For this review, take the finished solid that the model builds, in its own axes (mm). Face numbers are marked on the shaded views. A direction names the side the tool comes from. Round coordinates to 2 decimals unless told otherwise and drop trailing zeros. Write each loop counter-clockwise with the first axis right and the second up, starting at its lowest first coordinate (ties: lowest second). Pieces come first, ordered by that corner, then holes. Notation, with made-up numbers: M 28.5,49.5 L 78.5,49.5 A20 cw 78.5,88.5 Z; hole C 0,-24.75 d9. An arc over 180 degrees is marked long. Answer in a Markdown table with one row per item.
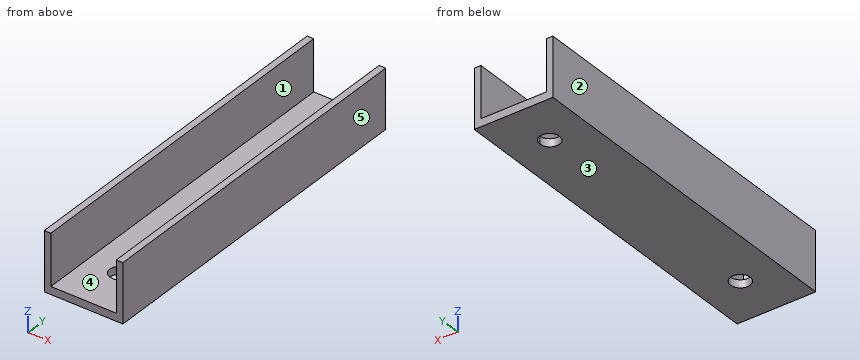
```python
from build123d import *

# Parameters (mm, degrees)
F0_R     = 3.175
F1_DEPTH = 19.05
F2_W     = 21.134718
F2_H     = 23.147546
F3_DEPTH = 140.54349


with BuildPart() as f1:
    # F0 (on Top) → F1 (new body)
    with BuildSketch(Plane.XY):
        with BuildLine():
            ThreePointArc((3.175, 41.452094), (2.245064, 43.697158), (0, 44.627094))
            ThreePointArc((0, 44.627094), (-2.245064, 39.20703), (3.175, 41.452094))
        make_face()
        Polygon((-12.7, -57.15), (12.7, -57.15), (12.7, 57.15), (0, 57.15), (-12.7, 57.15), align=None)
        with Locations((0, -41.452094)):
            Circle(F0_R, mode=Mode.SUBTRACT)
        with BuildLine():
            ThreePointArc((3.175, 41.452094), (-2.245064, 39.20703), (0, 44.627094))
            ThreePointArc((0, 44.627094), (2.245064, 43.697158), (3.175, 41.452094))
        make_face(mode=Mode.SUBTRACT)
    extrude(amount=F1_DEPTH)

    # F2 (on face) → F3 (cut)
    with BuildSketch(Plane(origin=(0, 57.15, 0), x_dir=(-1, 0, 0), z_dir=(0, 1, 0))):
        with Locations((0, 14.087191)):
            Rectangle(F2_W, F2_H)
    extrude(amount=-F3_DEPTH, mode=Mode.SUBTRACT)


solid = f1.part
```
Q1. Take a section at B-B (y = -6). State the section outline as (x, z) points, then the cut area to 3 significant figures.
Found:
| item | result |
|---|---|
| outline | M -12.7,0 L 12.7,0 L 12.7,19.05 L 10.57,19.05 L 10.57,2.51 L -10.57,2.51 L -10.57,19.05 L -12.7,19.05 Z |
| area | 134 mm² |
Q2. For probe 1 along Y at (x, z) = (0, 1.6); probe 2 along X at (y, z) = (23, 6.25); probe 3 along Z at (x, y) = (3.5, -1), list the stretches that pass through material, from the lowest coordinate up.
Found:
| item | result |
|---|---|
| probe 1 | -57.15 to -44.63, -38.28 to 38.28, 44.63 to 57.15 |
| probe 2 | -12.7 to -10.57, 10.57 to 12.7 |
| probe 3 | 0 to 2.51 |
Q3. Take a section at C-C (z = 1.5). State the section outline as (x, y) points (3 decimals), then the cut area to 3 significant figures.
Found:
| item | result |
|---|---|
| outline | M -12.7,-57.15 L 12.7,-57.15 L 12.7,57.15 L -12.7,57.15 Z; hole C 0,-41.452 d6.35; hole C 0,41.452 d6.35 |
| area | 2,840 mm² |
Q4. Machinability: for the marked faces 1 and 2, which of the approach directions +Z, -Z, +X, -X, +Y, -Y give a long, thin tool a straight path to every point of the face, cutting with its end or side? Answer none if there is none.
Found:
| item | result |
|---|---|
| face 1 | +Z, +Y, -Y |
| face 2 | +Z, -Z, -X, +Y, -Y |
Q5. Insertion check: P1, Ø10.5, axis at x = -2, y = -10, coming from the +Z side. The pin has a flat end and moves straight along its axis. Give the tip position at first contact, or say it passes through.
Found:
| item | result |
|---|---|
| P1 | z = 2.51 |
Q6. Take a section at D-D (x = -8). State the section outline as (y, z) points, then the cut area to 3 significant figures.
Found:
| item | result |
|---|---|
| outline | M -57.15,0 L 57.15,0 L 57.15,2.51 L -57.15,2.51 Z |
| area | 287 mm² |
Q7. Take a section at A-A (z = 7.5). State the section outline as (x, y) points.
Found:
| item | result |
|---|---|
| outline | M -12.7,-57.15 L -10.57,-57.15 L -10.57,57.15 L -12.7,57.15 Z; M 10.57,-57.15 L 12.7,-57.15 L 12.7,57.15 L 10.57,57.15 Z |
Q8. Mouldability with a two-part tool opening along X and no side actions: class the marked faces 3, 4 and 5 as +X half, -X half, draft (parallel to the pull), parting line (faces both ways), or undercut.
Found:
| item | result |
|---|---|
| face 3 | draft |
| face 4 | undercut |
| face 5 | +X half |
